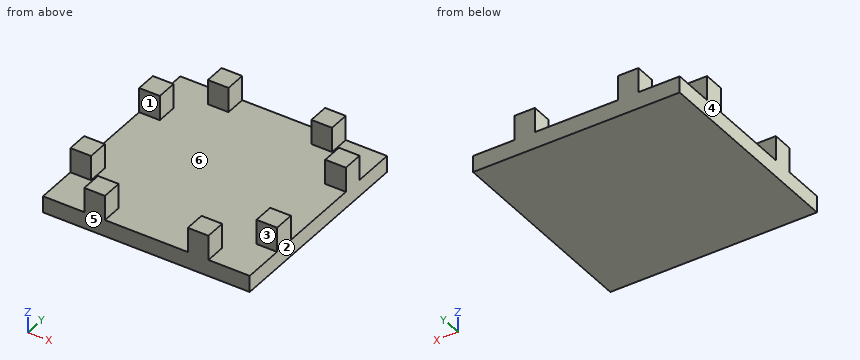
from build123d import *

# Parameters (mm, degrees)
F0_W     = 31.8008
F0_H     = 31.8008
F1_DEPTH = 2.54
F2_W     = 3.175
F2_H     = 3.175
F3_DEPTH = 3.81


with BuildPart() as f1:
    # F0 (on Top) → F1 (new body)
    with BuildSketch(Plane.XY):
        Rectangle(F0_W, F0_H)
    extrude(amount=-F1_DEPTH)

    # F2 (on Top) → F3 (join)
    with BuildSketch(Plane.XY):
        with Locations((-7.9629, 14.3129)):
            Rectangle(F2_W, F2_H)
        with Locations((-14.3129, 7.9629)):
            Rectangle(F2_W, F2_H)
        with Locations((14.3129, 7.9629)):
            Rectangle(F2_W, F2_H)
        with Locations((-14.3129, -7.9629)):
            Rectangle(F2_W, F2_H)
        with Locations((-7.9629, -14.3129)):
            Rectangle(F2_W, F2_H)
        with Locations((7.9629, 14.3129)):
            Rectangle(F2_W, F2_H)
        with Locations((14.3129, -7.9629)):
            Rectangle(F2_W, F2_H)
        with Locations((7.9629, -14.3129)):
            Rectangle(F2_W, F2_H)
    extrude(amount=F3_DEPTH)


solid = f1.part
Geometry: final body of the model. Coordinates: model frame, mm. Face numbers are marked on the shaded views. A direction names the side the tool comes from. Give positions to 0.01 mm unless a question says otherwise; leave off trailing zeros. Order: outer loops, then holes, each group sorted by start corner. A loop starts at its lowest first (then second) coordinate and runs counter-clockwise, first axis right, second up. Notation, with made-up numbers: (73, 65.5) -> (79, 65.5) arc R18 cw to (79, 71.5) -> close; hole circle Ø10 at (74, 89.5). An arc over 180 degrees is marked (long way). Put each result on its own line as item: value.
Q1. Pin query (flat end, axial travel): pin 1 (1 mm diameter, centred on y = -14.5, z = 1, fed in from -X); pin 2 (1.6 mm diameter, centred on y = -14.5, z = 2.5, fed in from +X); pin 3 (1.6 mm diameter, centred on x = 14, z = 2, fed in from -Y); pin 4 (1.5 mm diameter, centred on y = 3.5, z = 2, fed in from -X). Return the tip coordinate at first contact, or that it passes through.
Here are the results:
pin 1: stops at x = -9.55
pin 2: stops at x = 9.55
pin 3: stops at y = -9.55
pin 4: passes through
Q2. Section B-B, the plane x = -9. Return loops of the section in (y, z), then the cut area to 3 significant figures.
Here are the results:
outline: (-15.9, -2.54) -> (15.9, -2.54) -> (15.9, 3.81) -> (12.73, 3.81) -> (12.73, 0) -> (-12.73, 0) -> (-12.73, 3.81) -> (-15.9, 3.81) -> close
area: 105 mm^2
Q3. Section A-A, the plane z = 2.75. Count the separate pieces of the cut face and the enclosed holes in it, then the cut area to 3 significant figures.
Here are the results:
separate pieces: 8
enclosed holes: 0
area: 80.6 mm^2
Q4. Material intervals for L1, parallel to Y at x = -13.5, z = 1.5; L2, parallel to X at y = -9, z = 3, sorted ascending.
Here are the results:
L1: y = -9.55 to -6.38, 6.38 to 9.55
L2: x = -15.9 to -12.73, 12.73 to 15.9
Q5. Draft query along Y for the marked faces 4, 5 and 6. Return one class per face: released by +Y, released by -Y, zero draft, split by the parting line, or undercut.
Here are the results:
face 4: zero draft
face 5: released by -Y
face 6: undercut
Q6. Section D-D, the plane y = -10.5. Return loops of the section in (x, z), then the cut area to 3 significant figures.
Here are the results:
outline: (-15.9, -2.54) -> (15.9, -2.54) -> (15.9, 0) -> (-15.9, 0) -> close
area: 80.8 mm^2
Q7. Reachability of the marked faces 1, 2 and 3 from +Z, -Z, +X, -X, +Y, -Y: full face, straight path, thin tool, end or side. Return the list, or none.
Here are the results:
face 1: +Z, +X, -X
face 2: +Z, -Z, +X, +Y, -Y
face 3: +Z, +X, -X, -Y
